Input: part model. Units: mm. Frame: model coordinates. Face numbers are marked on the shaded views. A direction names the side the tool comes from. Round coordinates to 2 decimals unless told otherwise and drop trailing zeros. Order: outer loops, then holes, each group sorted by start corner. A loop starts at its lowest first (then second) coordinate and runs counter-clockwise, first axis right, second up. Notation, with made-up numbers: (0, 67) -> (35, 67) arc R7 cw to (35, 78) -> close; hole circle Ø11 at (16, -13.5). An arc over 180 degrees is marked (long way). Answer as CSV lines item,"result". Start each with the question number.
1) Line query: L1, parallel to X at y = 2.75, z = -23.5; L2, parallel to X at y = 3, z = -8; L3, parallel to Z at x = -2.25, y = 6. Output: solid intervals per line, ascending.
2) Section query B-B, the plane z = -23.5. Output: boundary loops of the cut face in (x, y).
3) First-contact query: P1, Ø1.6, axis at y = 9.5, z = -17, coming from the -X side; P2, Ø0.6, axis at x = 0, z = -33, coming from the +Y side; P3, Ø5, axis at x = -5, y = 7, coming from the -Z side. Flat tips, straight axial feed; report the tip coordinate or a pass-through.
4) Mould query, pull axis X, two halves, no side actions, for the marked faces 1, 2 and 3. Classes: +X half, -X half, draft (parallel to the pull), parting line (faces both ways), or undercut.
5) Section query C-C, the plane x = 7.75. Output: boundary loops of the cut face in (y, z), and give its area (3 significant figures).
6) Access query for the marked faces 4 and 5. Directions: +Z, -Z, +X, -X, +Y, -Y. A direction counts if a zero-diameter tool reaches every point of the face in a straight line with its end or side. Return the directions, or none.
7) Section query D-D, the plane z = -16.5. Output: boundary loops of the cut face in (x, y).
8) Section query A-A, the plane y = 4.5. Output: boundary loops of the cut face in (x, z).
```python
from build123d import *

# Parameters (mm, degrees)
SKETCH_1_R          = 2.5
EXTRUDE_1_DEPTH     = 9
SKETCH_3_W          = 2.5
SKETCH_3_H          = 3
EXTRUDE_2_DEPTH     = 1.5
CUT_EXTRUDE_1_REACH = 11
SKETCH_5_W          = 13
SKETCH_5_H          = 1.5
SKETCH_6_W          = 13
SKETCH_6_H          = 1.5
EXTRUDE_3_DEPTH     = 1
CUT_EXTRUDE_2_REACH = 35.5
SKETCH_7_W          = 13
SKETCH_7_H          = 1


with BuildPart() as part:
    # 草图1 → 凸台-拉伸1 (new body)
    with BuildSketch(Plane(origin=(0, 0, 0), x_dir=(1, 0, 0), z_dir=(0, 1, 0))):
        with BuildLine():
            Line((-2.382835885, 33.5), (8.617164115, 33.5))
            ThreePointArc((8.617164115, 33.5), (10.031377677, 32.914213562), (10.617164115, 31.5))
            Line((10.617164115, 31.5), (10.617164115, 2))
            ThreePointArc((10.617164115, 2), (10.031377677, 0.585786438), (8.617164115, 0))
            Line((8.617164115, 0), (0, 0))
            ThreePointArc((0, 0), (-5.710600422, 0.647655185), (-11.131122415, 2.557722132))
            ThreePointArc((-11.131122415, 2.557722132), (-12.111898361, 5.107720531), (-9.633282348, 6.257014206))
            ThreePointArc((-9.633282348, 6.257014206), (-8.243555708, 5.833986106), (-6.836394497, 5.473167269))
            ThreePointArc((-6.836394497, 5.473167269), (-5.139275919, 5.854675685), (-4.382835885, 7.421059613))
            Line((-4.382835885, 7.421059613), (-4.382835885, 31.5))
            ThreePointArc((-4.382835885, 31.5), (-3.797049447, 32.914213562), (-2.382835885, 33.5))
        make_face()
        with Locations((3.117164115, 23.5)):
            Circle(SKETCH_1_R, mode=Mode.SUBTRACT)
    extrude(amount=EXTRUDE_1_DEPTH)

    # 草图3 → 凸台-拉伸2 (add)
    with BuildSketch(Plane(origin=(0, 9, 0), x_dir=(1, 0, 0), z_dir=(0, 1, 0))):
        with Locations((-2.382835885, 17)):
            Rectangle(SKETCH_3_W, SKETCH_3_H)
        with Locations((8.617164115, 17)):
            Rectangle(SKETCH_3_W, SKETCH_3_H)
    extrude(amount=EXTRUDE_2_DEPTH)

    # 草图5 → 切除-拉伸1 (cut, up to next)
    with BuildSketch(Plane(origin=(0, 9, 0), x_dir=(1, 0, 0), z_dir=(0, 1, 0)), mode=Mode.PRIVATE) as cut_extrude_1_sk1:
        with Locations((2.117164115, 30.75)):
            Rectangle(SKETCH_5_W, SKETCH_5_H)
    cut_extrude_1_tool1 = extrude(cut_extrude_1_sk1.sketch, amount=-CUT_EXTRUDE_1_REACH, mode=Mode.PRIVATE) & part.part
    add(cut_extrude_1_tool1.solids().sort_by_distance((2.117164, 9, -30.75))[0], mode=Mode.SUBTRACT)

    # 草图6 → 凸台-拉伸3 (add)
    with BuildSketch(Plane(origin=(0, 9, 0), x_dir=(1, 0, 0), z_dir=(0, 1, 0))):
        with Locations((2.117164115, 30.75)):
            Rectangle(SKETCH_6_W, SKETCH_6_H)
    extrude(amount=-EXTRUDE_3_DEPTH)

    # 草图7 → 切除-拉伸2 (cut, up to next)
    with BuildSketch(Plane(origin=(0, 0, -33.5), x_dir=(-1, 0, 0), z_dir=(0, 0, -1)), mode=Mode.PRIVATE) as cut_extrude_2_sk1:
        with Locations((-2.117164115, 2)):
            Rectangle(SKETCH_7_W, SKETCH_7_H)
    cut_extrude_2_tool1 = extrude(cut_extrude_2_sk1.sketch, amount=-CUT_EXTRUDE_2_REACH, mode=Mode.PRIVATE) & part.part
    add(cut_extrude_2_tool1.solids().sort_by_distance((2.117164, 2, -33.5))[0], mode=Mode.SUBTRACT)


solid = part.part
```
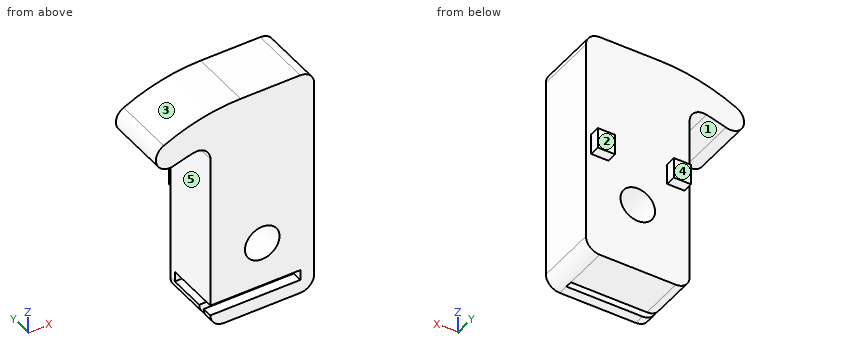
Findings:
1,L1,"x = -4.38 to 0.62, 5.62 to 10.62"
1,L2,"x = -4.38 to 10.62"
1,L3,"z = -33.5 to -31.5, -30 to -0.1"
2,outline,"(-4.38, 0) -> (0.62, 0) -> (0.62, 9) -> (-4.38, 9) -> close; (5.62, 0) -> (10.62, 0) -> (10.62, 9) -> (5.62, 9) -> close"
3,P1,"stops at x = -4.38"
3,P2,"stops at y = 9"
3,P3,"stops at z = -33.5"
4,face 1,"undercut"
4,face 2,"draft"
4,face 3,"-X half"
5,outline,"(0, -33.5) -> (1.5, -33.5) -> (1.5, -31.5) -> (0, -31.5) -> close; (0, -30) -> (8, -30) -> (8, -31.5) -> (2.5, -31.5) -> (2.5, -33.5) -> (9, -33.5) -> (9, -18.5) -> (10.5, -18.5) -> (10.5, -15.5) -> (9, -15.5) -> (9, 0) -> (0, 0) -> close"
5,area,"292 mm^2"
6,face 4,"+Z, -Z, +X, -X, +Y"
6,face 5,"-Z, -X, +Y, -Y"
7,outline,"(-4.38, 0) -> (10.62, 0) -> (10.62, 9) -> (9.87, 9) -> (9.87, 10.5) -> (7.37, 10.5) -> (7.37, 9) -> (-1.13, 9) -> (-1.13, 10.5) -> (-3.63, 10.5) -> (-3.63, 9) -> (-4.38, 9) -> close"
8,outline,"(-11.13, -2.56) arc R2 ccw to (-9.63, -6.26) arc R32.66 cw to (-6.84, -5.47) arc R2 cw to (-4.38, -7.42) -> (-4.38, -30) -> (8.62, -30) -> (8.62, -31.5) -> (-4.38, -31.5) arc R2 ccw to (-2.38, -33.5) -> (8.62, -33.5) arc R2 ccw to (10.62, -31.5) -> (10.62, -2) arc R2 ccw to (8.62, 0) -> (0, 0) arc R25.5 ccw to start; hole circle Ø5 at (3.12, -23.5)"
